Work out the finished part from the listing and answer in its coordinate system (mm). Face numbers are marked on the shaded views. A direction names the side the tool comes from. Round coordinates to 2 decimals unless told otherwise and drop trailing zeros. Loops run counter-clockwise (first coordinate to the right, second up) from the corner with the lowest first, then second, coordinate; pieces in that order, holes last.
Autodesk Inventor part; units mm, degrees
ref_plane "YZ Plane" through (0, 0, 0) normal (1, 0, 0) x (0, 1, 0)
ref_plane "XZ Plane" through (0, 0, 0) normal (0, 1, 0) x (-1, 0, 0)
ref_plane "XY Plane" through (0, 0, 0) normal (0, 0, 1) x (1, 0, 0)
sketch "Sketch1" plane through (0, 0, 0) normal (0, 0, 1) x (1, 0, 0)
  line L0 (0, 0) -> (25, 0)
  line L1 (25, 0) -> (25, 1.5)
  line L2 (25, 1.5) -> (0, 1.5)
  line L3 (0, 1.5) -> (0, 0)
  line L4 (0, 1.5) -> (1.5, 1.5)
  line L5 (1.5, 1.5) -> (1.5, 25)
  line L6 (1.5, 25) -> (0, 25)
  line L7 (0, 25) -> (0, 1.5)
  point P0 (1.5, 1.5)
  dimension "d0" = 25
  dimension "d1" = 1.5
  dimension "d2" = 25
extrude "Extrusion1" add sketch "Sketch1" along normal blind 15
sketch "Sketch2" plane through (0, 0, 0) normal (0, -1, 0) x (1, 0, 0)
  point P0 (0, 0)
  point P1 (12.5, 7.5)
  dimension "d5" = 12.5
  dimension "d6" = 7.5
hole "Hole1" at (12.5, 0, 7.5) direction (0, 1, 0) diameter 5 depth 8 tip angle 118
sketch "Sketch3" plane through (0, 0, 0) normal (-1, 0, 0) x (0, 0, 1)
  point P0 (0, 0)
  point P1 (7.5, 12.5)
  dimension "d14" = 12.5
  dimension "d15" = 7.5
hole "Hole2" at (0, 12.5, 7.5) direction (1, 0, 0) diameter 5 depth 8 tip angle 118
equation "\"d2\" = d0"
properties part number "25x25x25 Simple Angle Bracket"
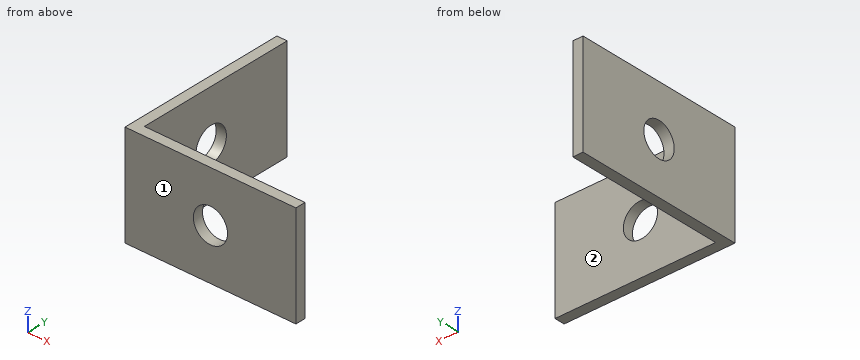
Item 1: For the marked faces 1 and 2, determine the directions among +Z, -Z, +X, -X, +Y, -Y from which every point of the face is accessible in a straight line to the end or side of a thin tool.
Item 2: Each of these flat-tipped pins is pushed along its axis until it touches: P1, Ø7.5, axis at y = 16.5, z = 8.5, coming from the +X side; P2, Ø3, axis at x = 12.5, z = 7.5, coming from the -Y side; P3, Ø7.5, axis at x = 13, z = 5.5, coming from the +Y side. Where does it stop, or does it pass through?
Item 3: Section C-C, the plane z = 7.5 is taken. Give the vertices of the cut face in (x, y).
Item 4: Section A-A, the plane x = 12.5 is taken. Give the vertices of the cut face in (y, z).
Item 5: Straight lines are drawn through the part: line 1 (Y direction, x = 0.6, z = 7.5); line 2 (Z direction, x = 12.5, y = 0.4). For each, find the intervals that lie inside material, in ascending order.
Item 6: Section D-D, the plane z = 2.75 is taken. Give the vertices of the cut face in (x, y).
Answer below:
1. face 1: +Z, -Z, +X, -X, -Y
1. face 2: +Z, -Z, +X, +Y
2. P1: stops at x = 1.5
2. P2: passes through
2. P3: stops at y = 1.5
3. outline: (0, 0) - (10, 0) - (10, 1.5) - (1.5, 1.5) - (1.5, 10) - (0, 10) - close; (0, 15) - (1.5, 15) - (1.5, 25) - (0, 25) - close; (15, 0) - (25, 0) - (25, 1.5) - (15, 1.5) - close
4. outline: (0, 0) - (1.5, 0) - (1.5, 5) - (0, 5) - close; (0, 10) - (1.5, 10) - (1.5, 15) - (0, 15) - close
5. line 1: y = 0 to 10, 15 to 25
5. line 2: z = 0 to 5, 10 to 15
6. outline: (0, 0) - (25, 0) - (25, 1.5) - (1.5, 1.5) - (1.5, 25) - (0, 25) - close
